Geometry: final body of the model. Coordinates: model frame, mm. A direction names the side the tool comes from. Round coordinates to 2 decimals unless told otherwise and drop trailing zeros. Loops run counter-clockwise (first coordinate to the right, second up) from the corner with the lowest first, then second, coordinate; pieces in that order, holes last. Notation, with made-up numbers: (57.5, 48) - (83.5, 48) arc R22 ccw to (83.5, 77) - close; hole circle Ø3 at (2, 49.5). An arc over 180 degrees is marked (long way). Write item = value, one per line. Start each with the question number.
Item 1: First-contact query: pin 1 (6 mm diameter, centred on x = 3.5, y = 3.5, fed in from +Z); pin 2 (5 mm diameter, centred on x = 4.5, z = -8, fed in from -Y); pin 3 (1 mm diameter, centred on y = 0.5, z = 42.5, fed in from -X); pin 4 (5 mm diameter, centred on y = 4, z = 46, fed in from -X). Flat tips, straight axial feed; report the tip coordinate or a pass-through.
Item 2: Line query: line 1 (Z direction, x = -1, y = -2.5); line 2 (Z direction, x = 1.5, y = -4.75); line 3 (X direction, y = -1.5, z = 57). Output: solid intervals per line, ascending. Write a range as from..to.
Item 3: Section A-A (x = 0). Return loops of the section in (y, z), plus the area to 3 significant figures.
Item 4: Section D-D (z = 16). Return loops of the section in (x, y).
Item 5: Section C-C (z = -3). Return loops of the section in (x, y), plus the area to 3 significant figures.
Item 6: Access query for faces 1 (the flat face through (2, 2, 46)), 2 (the cylindrical face through (-6, 0, 15)), 3 (the cylindrical face through (3, 0, -18)), 4 (the cylindrical face through (-3, 0, 53)). Directions: +Z, -Z, +X, -X, +Y, -Y. A direction counts if a zero-diameter tool reaches every point of the face in a straight line with its end or side. Return the directions, or none.
Item 7: Draft query along Z for faces 5 (the flat face through (-3, -1, 0)), 6 (the cylindrical face through (0.54, -2.44, 45.65)), 7 (the cylindrical face through (-3, 0, 38)). Return one class per face: pulls with the +Z half, pulls with the -Z half, needs draft (parallel to the pull), parting line crosses it, or undercut.
from build123d import *

# Parameters (mm, degrees)
SKETCH_1_R          = 6
EXTRUDE_1_DEPTH     = 30
SKETCH_2_R          = 3
EXTRUDE_2_DEPTH     = 20
SKETCH_3_R          = 3
EXTRUDE_3_DEPTH     = 30
SKETCH_4_R          = 6.707362288
SKETCH_4_R_2        = 2.5
CUT_EXTRUDE_1_DEPTH = 0.7
SKETCH_5_R          = 8.291110755
SKETCH_5_R_2        = 2.5
CUT_EXTRUDE_2_DEPTH = 0.7


with BuildPart() as part:
    # 草图1 → 凸台-拉伸1 (new body)
    with BuildSketch(Plane.XY):
        Circle(SKETCH_1_R)
    extrude(amount=EXTRUDE_1_DEPTH)

    # 草图2 → 凸台-拉伸2 (add)
    with BuildSketch(Plane(origin=(0, 0, 0), x_dir=(-1, 0, 0), z_dir=(0, 0, -1))):
        Circle(SKETCH_2_R)
    extrude(amount=EXTRUDE_2_DEPTH)

    # 草图3 → 凸台-拉伸3 (add)
    with BuildSketch(Plane.XY.offset(30)):
        Circle(SKETCH_3_R)
    extrude(amount=EXTRUDE_3_DEPTH)

    # 草图4 → 切除-拉伸1 (cut)
    with BuildSketch(Plane(origin=(0, 0, -16), x_dir=(-1, 0, 0), z_dir=(0, 0, -1))):
        Circle(SKETCH_4_R)
        Circle(SKETCH_4_R_2, mode=Mode.SUBTRACT)
    extrude(amount=-CUT_EXTRUDE_1_DEPTH, mode=Mode.SUBTRACT)

    # 草图5 → 切除-拉伸2 (cut)
    with BuildSketch(Plane(origin=(0, 0, 45.3), x_dir=(-1, 0, 0), z_dir=(0, 0, -1))):
        Circle(SKETCH_5_R)
        Circle(SKETCH_5_R_2, mode=Mode.SUBTRACT)
    extrude(amount=-CUT_EXTRUDE_2_DEPTH, mode=Mode.SUBTRACT)


solid = part.part
Taken from the geometry:
q1.pin_1 = 60
q1.pin_2 = -2.24
q1.pin_3 = -3
q1.pin_4 = -2.6
q2.line_1 = -20..-16, -15.3..45.3, 46..60
q2.line_2 = 0..30
q2.line_3 = -2.6..2.6
q3.outline = (-6, 0) - (-3, 0) - (-3, -15.3) - (-2.5, -15.3) - (-2.5, -16) - (-3, -16) - (-3, -20) - (3, -20) - (3, -16) - (2.5, -16) - (2.5, -15.3) - (3, -15.3) - (3, 0) - (6, 0) - (6, 30) - (3, 30) - (3, 45.3) - (2.5, 45.3) - (2.5, 46) - (3, 46) - (3, 60) - (-3, 60) - (-3, 46) - (-2.5, 46) - (-2.5, 45.3) - (-3, 45.3) - (-3, 30) - (-6, 30) - close
q3.area = 659 mm^2
q4.outline = circle Ø12 at (0, 0)
q5.outline = circle Ø6 at (0, 0)
q5.area = 28.3 mm^2
q6.face_1 = none
q6.face_2 = +Z, -Z
q6.face_3 = -Z
q6.face_4 = +Z
q7.face_5 = pulls with the -Z half
q7.face_6 = undercut
q7.face_7 = needs draft
